Drawing for the job (mm, zero at the part's lowest x, y, z). A direction names the side the tool comes from. Round coordinates to 2 decimals unless told otherwise and drop trailing zeros. Loops run counter-clockwise (first coordinate to the right, second up) from the corner with the lowest first, then second, coordinate; pieces in that order, holes last. Notation, with made-up numbers: (83.5, -16) - (125.5, -16) arc R17 ccw to (125.5, 17) - close; hole circle Ø2 at (-11, 77.5). An arc over 180 degrees is marked (long way). Put each result on its own line as item: value.
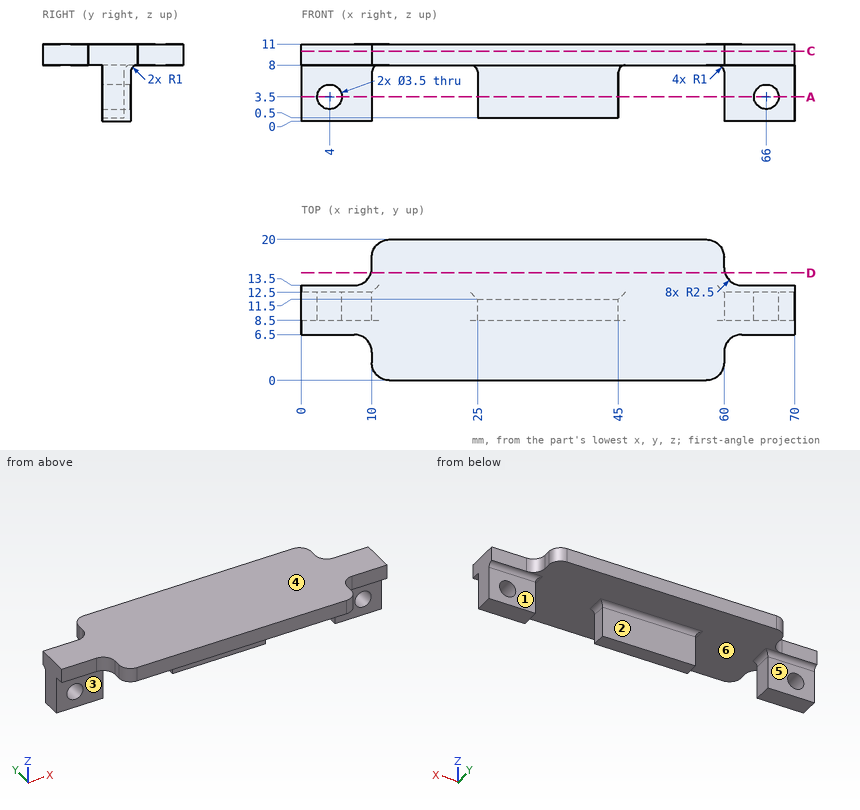
1. Probe line 1 along X through (y, z) = (10.75, 3.5); line 2 along Z through (x, y) = (66, 10.1); line 3 along Z through (x, y) = (16, 9). List the from-to ranges inside material, lowest first. Write a range as [from, to].
A:
line 1: x = [0, 2.25], [5.75, 10], [25, 45], [60, 64.25], [67.75, 70]
line 2: z = [0, 1.75], [5.25, 11]
line 3: z = [8, 11]
2. Band-saw the part on D-D (y = 15.25). List the corners of the cut face in (x, z) (3 decimals).
A:
outline: (9.885, 8) - (60.115, 8) - (60.115, 11) - (9.885, 11) - close
3. Tool access for the marked faces 3, 4, 5 and 6: list every direction of +Z, -Z, +X, -X, +Y, -Y with a clear straight run to the whole face (end or side of a thin tool).
A:
face 3: -Z, +X, -X, -Y
face 4: +Z, +X, -X, +Y, -Y
face 5: -Z, +X, -X, +Y
face 6: -Z
4. Band-saw the part on C-C (z = 10). List the corners of the cut face in (x, y), plus the area to 3 significant figures.
A:
outline: (0, 6.5) - (7.5, 6.5) arc R2.5 cw to (10, 4) - (10, 2.5) arc R2.5 ccw to (12.5, 0) - (57.5, 0) arc R2.5 ccw to (60, 2.5) - (60, 4) arc R2.5 cw to (62.5, 6.5) - (70, 6.5) - (70, 13.5) - (62.5, 13.5) arc R2.5 cw to (60, 16) - (60, 17.5) arc R2.5 ccw to (57.5, 20) - (12.5, 20) arc R2.5 ccw to (10, 17.5) - (10, 16) arc R2.5 cw to (7.5, 13.5) - (0, 13.5) - close
area: 1,140 mm²
5. Pin check, flat tips, straight feed: P1, Ø1.5, axis at x = 67, z = 10, coming from the -Y side; P2, Ø1.6, axis at y = 17, z = 10, coming from the +X side; P3, Ø10, axis at x = 21.5, y = 7, coming from the -Z side. Stop position of each tip, or through.
A:
P1: stops at y = 6.5
P2: stops at x = 60
P3: stops at z = 0.5
6. Two-plate mould, pull along X, no slides. Class the marked faces 1 and 2: pulls with the +X half, pulls with the -X half, needs draft (parallel to the pull), parting line crosses it, or undercut.
A:
face 1: needs draft
face 2: undercut
7. Band-saw the part on A-A (z = 3.5). List the corners of the cut face in (x, y), plus the area to 3 significant figures.
A:
outline: (0, 8.5) - (2.25, 8.5) - (2.25, 12.5) - (0, 12.5) - close; (5.75, 8.5) - (10, 8.5) - (10, 12.5) - (5.75, 12.5) - close; (25, 8.5) - (45, 8.5) - (45, 11.5) - (25, 11.5) - close; (60, 8.5) - (64.25, 8.5) - (64.25, 12.5) - (60, 12.5) - close; (67.75, 8.5) - (70, 8.5) - (70, 12.5) - (67.75, 12.5) - close
area: 112 mm²
